```python
from build123d import *

# Parameters (mm, degrees)
PAD_DEPTH          = 5
POLARPATTERN_COUNT = 8


with BuildPart() as part:
    # Sketch → Pad (new body)
    with BuildSketch(Plane.XY):
        with BuildLine():
            ThreePointArc((0.451745, 0.892147), (0.075949, 0.997112), (-0.311411, 0.950275))
            Line((-0.435975, 1.330386), (-0.311411, 0.950275))
            Line((-0.348532, 2.282026), (-0.435975, 1.330386))
            ThreePointArc((0.348532, 2.282026), (0, 2.6), (-0.348532, 2.282026))
            Line((0.348532, 2.282026), (0.435975, 1.330386))
            ThreePointArc((0.632444, 1.249006), (0.535757, 1.293431), (0.435975, 1.330386))
            Line((0.632444, 1.249006), (0.451745, 0.892147))
        make_face()
    pad = extrude(amount=PAD_DEPTH)

    # PolarPattern: Pad ×8 about axis
    polarpattern_axis = Axis((0, 0, 0), (0, 0, 1))
    for i in range(1, POLARPATTERN_COUNT):
        add(pad.rotate(polarpattern_axis, i * 360 / POLARPATTERN_COUNT))


solid = part.part
```
The listing builds one solid part. Answer for the finished solid, in the listing's coordinates (mm). A direction names the side the tool comes from. Give positions to 0.01 mm unless a question says otherwise; leave off trailing zeros. Write each loop counter-clockwise with the first axis right and the second up, starting at its lowest first coordinate (ties: lowest second). Pieces come first, ordered by that corner, then holes. Notation, with made-up numbers: (10.25, 37) -> (58.25, 37) arc R30 ccw to (58.25, 59) -> close; hole circle Ø11 at (74.25, -27.75). An arc over 180 degrees is marked (long way). Use one line per item in the form item = value.
1) Section B-B on y = -0.15 is taken. Write down the section's boundary in (x, z).
Result:
outline = (-2.57, 0) -> (-0.99, 0) -> (-0.99, 5) -> (-2.57, 5) -> close; (0.99, 0) -> (2.57, 0) -> (2.57, 5) -> (0.99, 5) -> close
2) For a pull along X with two mould halves and no side action, classify faces 5 (the flat face through (-1.81, -0.39, 2.46)), 6 (the flat face through (0.39, 1.81, 2.46)), 7 (the flat face through (-1, -1, 5)) as +X half, -X half, draft (parallel to the pull), parting line (faces both ways), or undercut.
Result:
face_5 = -X half
face_6 = undercut
face_7 = draft
3) Section A-A on x = 1.75 is taken. Write down the section's boundary in (y, z).
Result:
outline = (-1.9, 0) -> (-1.23, 0) -> (-1.23, 5) -> (-1.9, 5) -> close; (-0.4, 0) -> (0.4, 0) -> (0.4, 5) -> (-0.4, 5) -> close; (1.23, 0) -> (1.9, 0) -> (1.9, 5) -> (1.23, 5) -> close
4) A tool of negligible diameter and unlimited length cuts with its end or side. For faces 1 (the flat face through (0.39, -1.81, 2.46)), 2 (the flat face through (1.81, -0.39, 2.46)), 3 (the flat face through (-1.81, 0.39, 2.46)), 4 (the flat face through (-0.39, 1.81, 2.46)), from which of +Z, -Z, +X, -X, +Y, -Y can it reach the whole face along a straight path? Write none if from no direction.
Result:
face_1 = +Z, -Z, -Y
face_2 = +Z, -Z, +X
face_3 = +Z, -Z, -X
face_4 = +Z, -Z, +Y
5) Section C-C on x = -0.1 is taken. Write down the section's boundary in (y, z).
Result:
outline = (-2.59, 0) -> (-0.99, 0) -> (-0.99, 5) -> (-2.59, 5) -> close; (0.99, 0) -> (2.59, 0) -> (2.59, 5) -> (0.99, 5) -> close
6) Straight lines are drawn through the part: probe 1 along Y at (x, z) = (-1.55, 2); probe 2 along Y at (x, z) = (-1.4, 3.85); probe 3 along X at (y, z) = (1.45, 2.6). For each, find the intervals that lie inside material, in ascending order.
Result:
probe_1 = -1.94 to -0.99, -0.42 to 0.42, 0.99 to 1.94
probe_2 = -1.88 to -0.81, -0.43 to 0.43, 0.81 to 1.88
probe_3 = -1.91 to -0.87, -0.42 to 0.42, 0.87 to 1.91
7) Each of these flat-tipped pins is pushed along its axis until it touches: P1, Ø1, axis at x = -0.5, z = 4, coming from the -Y side; P2, Ø1, axis at y = -1, z = 4, coming from the +X side; P3, Ø2, axis at x = 1.5, z = 4, coming from the +Y side. Where does it stop, or does it pass through?
Result:
P1 = -2.6
P2 = 1.93
P3 = 1.94
8) Section D-D on x = -1.55 is taken. Write down the section's boundary in (y, z).
Result:
outline = (-1.94, 0) -> (-0.99, 0) -> (-0.99, 5) -> (-1.94, 5) -> close; (-0.42, 0) -> (0.42, 0) -> (0.42, 5) -> (-0.42, 5) -> close; (0.99, 0) -> (1.94, 0) -> (1.94, 5) -> (0.99, 5) -> close
